from build123d import *

# Parameters (mm, degrees)
BOSS_EXTRUDE1_DEPTH = 5.08
SKETCH3_W           = 4.826
SKETCH3_H           = 8.41502
SKETCH3_W_2         = 6.35
SKETCH3_H_2         = 5.08
CUT_EXTRUDE1_DEPTH  = 6.0800001


with BuildPart() as part:
    # Sketch2 → Boss-Extrude1 (new body)
    with BuildSketch(Plane.XY):
        with BuildLine():
            Line((190.5, 0.24003), (190.5, -0.24003))
            add(Edge.make_bspline(
                [(47.625, -11.59002), (49.21258277, -11.573232478), (52.324251607, -11.529902789), (58.609790093, -11.383526435), (66.486474066, -11.388894153), (76.012099473, -11.081769852), (85.601411445, -10.666111308), (95.189705286, -10.104719356), (104.778286225, -9.448700637), (114.303143312, -8.704754793), (123.828345261, -7.885794466), (133.353195338, -6.990482738), (142.87823509, -6.029908512), (152.403404308, -5.006647903), (161.928923416, -3.922089872), (171.454029858, -2.768063081), (180.980468385, -1.553123331), (187.325723566, -0.677879401), (190.5, -0.24003)],
                knots=[0.63243392, 0.63243392, 0.63243392, 0.63243392, 0.644639622, 0.656358033, 0.680768177, 0.705187031, 0.729619522, 0.754557907, 0.779023814, 0.803506448, 0.828005419, 0.852521438, 0.877054004, 0.901603249, 0.92617022, 0.95075713, 0.975365769, 1, 1, 1, 1], degree=3))
            Line((47.625, -11.59002), (47.625, 11.59002))
            add(Edge.make_bspline(
                [(190.5, 0.24003), (187.325723566, 0.677879401), (180.980468385, 1.553123331), (171.454029858, 2.768063081), (161.928923416, 3.922089872), (152.403404308, 5.006647903), (142.87823509, 6.029908512), (133.353195338, 6.990482738), (123.828345261, 7.885794466), (114.303143312, 8.704754793), (104.778286225, 9.448700637), (95.189705286, 10.104719356), (85.601411445, 10.666111308), (76.012099473, 11.081769852), (66.486474066, 11.388894153), (58.609790093, 11.383526435), (52.324251607, 11.529902789), (49.21258277, 11.573232478), (47.625, 11.59002)],
                knots=[0, 0, 0, 0, 0.024634231, 0.04924287, 0.07382978, 0.098396751, 0.122945996, 0.147478562, 0.171994581, 0.196493552, 0.220976186, 0.245442093, 0.270380478, 0.294812969, 0.319231823, 0.343641967, 0.355360378, 0.36756608, 0.36756608, 0.36756608, 0.36756608], degree=3))
        make_face()
    extrude(amount=BOSS_EXTRUDE1_DEPTH)

    # Sketch3 → Cut-Extrude1 (cut, through all)
    with BuildSketch(Plane(origin=(0, 0, 0), x_dir=(-1, 0, 0), z_dir=(0, 0, -1))):
        with Locations((-50.038, -7.38251)):
            Rectangle(SKETCH3_W, SKETCH3_H)
        with Locations((-50.038, 7.38251)):
            Rectangle(SKETCH3_W, SKETCH3_H)
        with Locations((-68.326, 0)):
            Rectangle(SKETCH3_W_2, SKETCH3_H_2)
    extrude(amount=-CUT_EXTRUDE1_DEPTH, mode=Mode.SUBTRACT)


solid = part.part
Source: CAD feature listing. Evaluate the final solid. Frame: model axes, mm. A direction names the side the tool comes from. Coordinates: 2 decimals unless noted, no trailing zeros. Answer in a Markdown table with one row per item.
Q1. First-contact query: pin 1 (3 mm diameter, centred on y = 6.5, z = 1, fed in from -X). Flat tip, straight axial feed; report the tip coordinate or a pass-through.
Answers below:
| item | result |
|---|---|
| pin 1 | stops at x = 52.45 |
Q2. Ray query, probe 1 along X at (y, z) = (0, 2.1) (3 decimals); probe 2 along Y at (x, z) = (164, 3.45); probe 3 along Y at (x, z) = (131.5, 1.7). Return the intervals inside material, ascending. Write a range as from..to.
Answers below:
| item | result |
|---|---|
| probe 1 | x = 47.625..65.151, 71.501..190.5 |
| probe 2 | y = -3.67..3.67 |
| probe 3 | y = -7.16..7.16 |
Q3. Draft query along X for faces 1 (the flat face through (71.501, 0, 3)), 2 (the flat face through (50, -3.175, 3)), 3 (the flat face through (52.451, 7, 3)). Return one class per face: pulls with the +X half, pulls with the -X half, needs draft (parallel to the pull), parting line crosses it, or undercut.
Answers below:
| item | result |
|---|---|
| face 1 | undercut |
| face 2 | needs draft |
| face 3 | pulls with the -X half |
Q4. Set-up query: faces 4 (the flat face through (52.451, -7, 3)), 5 (the flat face through (104, 0, 0)), 6 (the flat face through (68, -2.54, 3)), 7 (the flat face through (50, 3.175, 3)). Return all of +Z, -Z, +X, -X, +Y, -Y with unobstructed straight access to the full face (end or side cutting, diameter ignored); none if empty.
Answers below:
| item | result |
|---|---|
| face 4 | +Z, -Z, -X, -Y |
| face 5 | -Z, +X, -X, +Y, -Y |
| face 6 | +Z, -Z |
| face 7 | +Z, -Z, -X, +Y |
